Can you work these out from the drawing? Everything is in mm from the part's minimum corner. A direction names the side the tool comes from. Round coordinates to 2 decimals unless told otherwise and drop trailing zeros. Order: outer loops, then holes, each group sorted by start corner. A loop starts at its lowest first (then second) coordinate and runs counter-clockwise, first axis right, second up. Notation, with made-up numbers: M 45.5,-39 L 90.5,-39 A25 ccw 90.5,-25 Z; hole C -33,26 d4. An arc over 180 degrees is marked long. Answer as CSV lines item,"result". Start each with the question number.
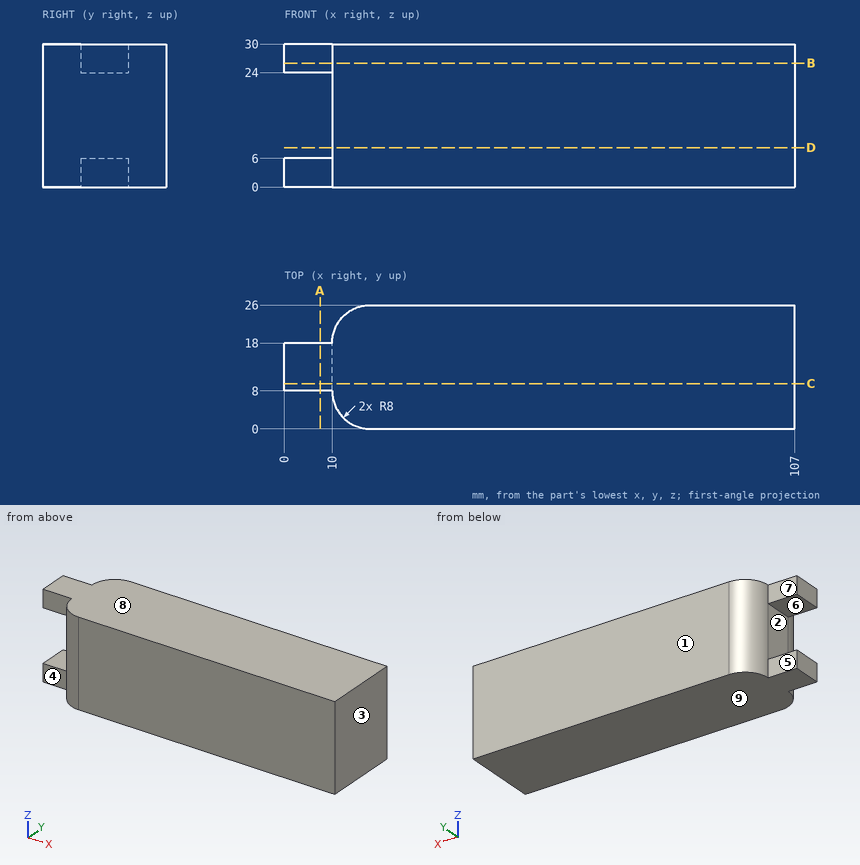
(1) I want a section at C-C on y = 9.5. Write out the boundary of the cut face in (x, z), and give its area (3 significant figures).
(2) If we mould it in two halves opening along Z, with no side actions, what happens to the marked faces 6, 7, 8 and 9? For each: +Z half, -Z half, draft (parallel to the pull), parting line (faces both ways), or undercut.
(3) I want a section at B-B on z = 26. Write out the boundary of the cut face in (x, y), and give its area (3 significant figures).
(4) I want a section at D-D on z = 8.25. Write out the boundary of the cut face in (x, y), and give its area (3 significant figures).
(5) For the marked faces 1, 2, 3, 4 and 5, which set-ups out of +Z, -Z, +X, -X, +Y, -Y let a thin tool reach every point of the face, with its end or its side?
(6) I want a section at A-A on x = 7.5. Write out the boundary of the cut face in (y, z), and give its area (3 significant figures).
(7) I'm going to push flat-ended pins straight in: P1, Ø1, axis at y = 3, z = 26.5, coming from the -X side; P2, Ø3, axis at x = 14.5, z = 4.5, coming from the +Y side; P3, Ø4, axis at y = 16.5, z = 13.5, coming from the -X side. Where does each tip first touch, or does it pass through?
(8) If I drill on line 1 along Z through (x, y) = (6, 11); line 2 along X through (y, z) = (13.25, 6.5); line 3 along X through (y, z) = (3.75, 27.5), over which ranges is the centre line in solid material (lowest first)?
From the geometry:
1,outline,"M 0,0 L 107,0 L 107,30 L 0,30 L 0,24 L 10,24 L 10,6 L 0,6 Z"
1,area,"3,030 mm²"
2,face 6,"undercut"
2,face 7,"draft"
2,face 8,"+Z half"
2,face 9,"-Z half"
3,outline,"M 0,8 L 10,8 A8 ccw 18,0 L 107,0 L 107,26 L 18,26 A8 ccw 10,18 L 0,18 Z"
3,area,"2,590 mm²"
4,outline,"M 10,8 A8 ccw 18,0 L 107,0 L 107,26 L 18,26 A8 ccw 10,18 Z"
4,area,"2,490 mm²"
5,face 1,"+Z, -Z, +X, -X, +Y"
5,face 2,"-X, +Y, -Y"
5,face 3,"+Z, -Z, +X, +Y, -Y"
5,face 4,"+Z, -Z, -X, -Y"
5,face 5,"+Z, -Z, -X, +Y"
6,outline,"M 8,0 L 18,0 L 18,6 L 8,6 Z; M 8,24 L 18,24 L 18,30 L 8,30 Z"
6,area,"120 mm²"
7,P1,"x = 11.39"
7,P2,"y = 25.75"
7,P3,"x = 10"
8,line 1,"0 to 6, 24 to 30"
8,line 2,"10 to 107"
8,line 3,"11.22 to 107"
